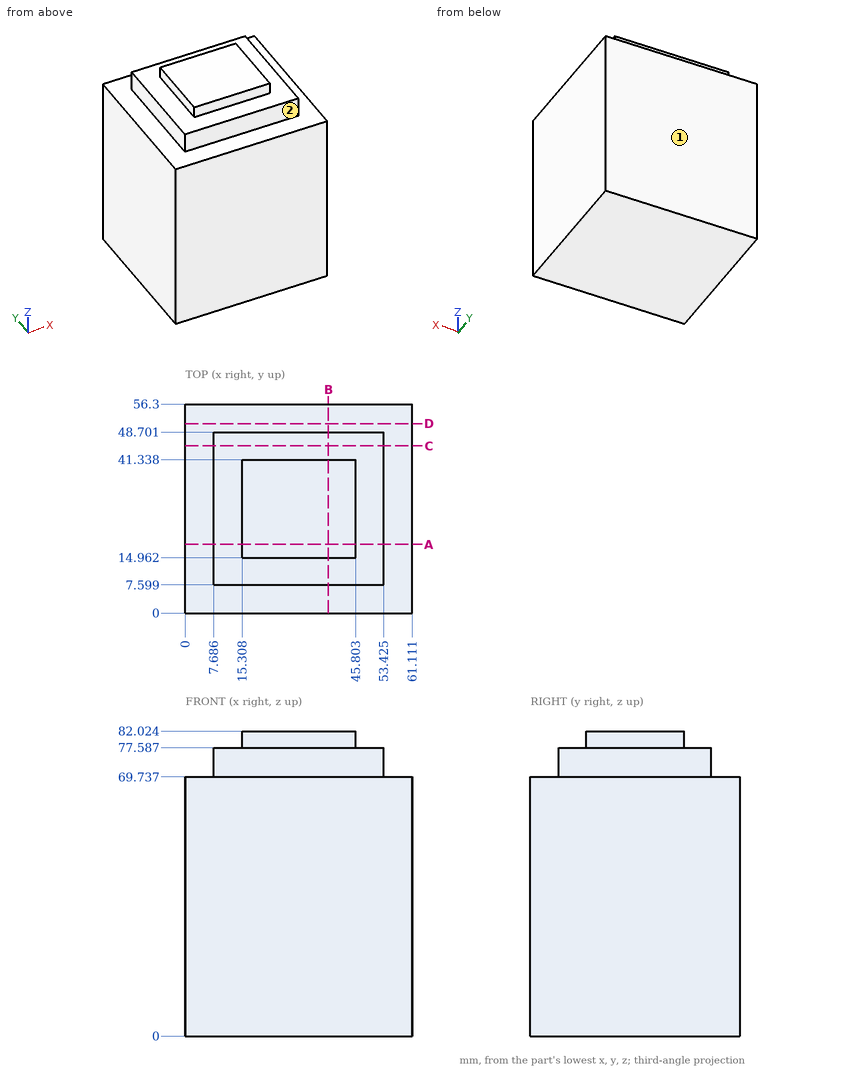
Input: dimensioned drawing with shaded views. Units: mm. Origin: part minimum x, y, z. A direction names the side the tool comes from. Coordinates: 2 decimals unless noted, no trailing zeros. Loops run counter-clockwise (first coordinate to the right, second up) from the corner with the lowest first, then second, coordinate; pieces in that order, holes last. Notation, with made-up numbers: (2, 23) -> (29, 23) arc R21 ccw to (29, 34) -> close; hole circle Ø11 at (23.25, 63.5). An arc over 180 degrees is marked (long way). One line per item, written item: value. Start each with the question number.
Q1. Section query D-D, the plane y = 51. Return the cut outline in (x, z).
Q2. Section query B-B, the plane x = 38.5. Return the cut outline in (y, z).
Q3. Line query: line 1 along Z through (x, y) = (5, 46); line 2 along X through (y, z) = (18.5, 70.5) (1 decimal); line 3 along Z through (x, y) = (28.5, 42.5). Output: solid intervals per line, ascending.
Q4. Section query A-A, the plane y = 18.5. Return the cut outline in (x, z) (1 decimal), and give its area (3 significant figures).
Q5. Contact query for flat-ended pins moving along their axis: P1, Ø1.3, axis at y = 29, z = 80.5, coming from the -X side; P2, Ø3.5, axis at x = 26.5, z = 79, coming from the +Y side; P3, Ø2, axis at x = 49.5, y = 48.5, coming from the +Z side. Output: stop coordinate, or through.
Q6. Section query C-C, the plane y = 45. Return the cut outline in (x, z) (1 decimal).
Q7. Set-up query: the marked faces 1 and 2. Return all of +Z, -Z, +X, -X, +Y, -Y with unobstructed straight access to the full face (end or side cutting, diameter ignored); none if empty.
Results:
1. outline: (0, 0) -> (61.11, 0) -> (61.11, 69.74) -> (0, 69.74) -> close
2. outline: (0, 0) -> (56.3, 0) -> (56.3, 69.74) -> (48.7, 69.74) -> (48.7, 77.59) -> (41.34, 77.59) -> (41.34, 82.02) -> (14.96, 82.02) -> (14.96, 77.59) -> (7.6, 77.59) -> (7.6, 69.74) -> (0, 69.74) -> close
3. line 1: 0 to 69.74
3. line 2: 7.7 to 53.4
3. line 3: 0 to 77.59
4. outline: (0, 0) -> (61.1, 0) -> (61.1, 69.7) -> (53.4, 69.7) -> (53.4, 77.6) -> (45.8, 77.6) -> (45.8, 82) -> (15.3, 82) -> (15.3, 77.6) -> (7.7, 77.6) -> (7.7, 69.7) -> (0, 69.7) -> close
4. area: 4,760 mm^2
5. P1: x = 15.31
5. P2: y = 48.7
5. P3: z = 77.59
6. outline: (0, 0) -> (61.1, 0) -> (61.1, 69.7) -> (53.4, 69.7) -> (53.4, 77.6) -> (7.7, 77.6) -> (7.7, 69.7) -> (0, 69.7) -> close
7. face 1: +Z, -Z, +X, -X, +Y
7. face 2: +Z, +X, -X, -Y
